```python
from build123d import *

# Parameters (mm, degrees)
CUT_EXTRUDE1_START        = 15
CUT_EXTRUDE1_DEPTH        = 10.5
CUT_EXTRUDE1_START_2      = 25.5
CUT_EXTRUDE1_2_DEPTH      = 4
CUT_EXTRUDE1_START_3      = -5
CUT_EXTRUDE1_3_DEPTH      = 3.568757805
BOSS_EXTRUDE1_DEPTH       = 0.5
BOSS_EXTRUDE2_DEPTH       = 0.5
SKETCH4_W                 = 14.5
SKETCH4_H                 = 15
CUT_EXTRUDE2_DEPTH        = 10.672144385
BOSS_EXTRUDE3_DEPTH       = 10.5
F_3_CLEARANCE_HOLE1_D     = 2.9
F_3_CLEARANCE_HOLE1_DEPTH = 6.031783808


with BuildPart() as part:
    # Cut-Extrude1: read off the stored shape, not the designer's step
    # Cut-Extrude1 outline → Cut-Extrude1 (new body)
    with BuildSketch(Plane.XY.offset(CUT_EXTRUDE1_START)):
        with BuildLine():
            Line((337.250458866, -1.431242195), (336.422603251, -1.431242195))
            Line((336.422603251, -1.431242195), (336.422603251, 13.568757805))
            Line((336.422603251, 13.568757805), (323.834138276, 13.568757805))
            Line((323.834138276, 13.568757805), (323.608997572, 10.166078708))
            ThreePointArc((323.608997572, 10.166078708), (323.181382472, 9.560091757), (322.443572772, 9.635667582))
            Line((322.443572772, 9.635667582), (321.491292518, 10.587947835))
            ThreePointArc((321.491292518, 10.587947835), (321.1243382, 10.696161689), (320.834327975, 10.446642593))
            ThreePointArc((320.834327975, 10.446642593), (320.5127775, 9.115460329), (320.529645575, 7.746096829))
            ThreePointArc((320.529645575, 7.746096829), (320.552977781, 7.656046386), (320.596479116, 7.57382043))
            ThreePointArc((320.596479116, 7.57382043), (320.51875348, 5.851708999), (319.722869168, 4.322566357))
            ThreePointArc((319.722869168, 4.322566357), (320.011740784, 3.764617073), (320.636356902, 3.832506086))
            Line((320.636356902, 3.832506086), (321.56122175, 4.617919231))
            ThreePointArc((321.56122175, 4.617919231), (322.32777998, 4.668660807), (322.750458866, 4.027155713))
            Line((322.750458866, 4.027155713), (322.750458866, -4.431242195))
            Line((322.750458866, -4.431242195), (342.750458866, -4.431242195))
            Line((342.750458866, -4.431242195), (342.750458866, -2.431242195))
            Line((342.750458866, -2.431242195), (338.250458866, -2.431242195))
            Line((338.250458866, -2.431242195), (337.250458866, -1.431242195))
        make_face()
    extrude(amount=CUT_EXTRUDE1_DEPTH)

    # Cut-Extrude1 2 outline → Cut-Extrude1 2 (add)
    with BuildSketch(Plane.XY.offset(CUT_EXTRUDE1_START_2)):
        with BuildLine():
            Line((337.250458866, -1.431242195), (336.422603251, -1.431242195))
            Line((336.422603251, -1.431242195), (336.422603251, 13.568757805))
            Line((336.422603251, 13.568757805), (323.834138276, 13.568757805))
            Line((323.834138276, 13.568757805), (323.608997572, 10.166078708))
            ThreePointArc((323.608997572, 10.166078708), (323.181382472, 9.560091757), (322.443572772, 9.635667582))
            Line((322.443572772, 9.635667582), (321.491292518, 10.587947835))
            ThreePointArc((321.491292518, 10.587947835), (321.1243382, 10.696161689), (320.834327975, 10.446642593))
            ThreePointArc((320.834327975, 10.446642593), (320.5127775, 9.115460329), (320.529645575, 7.746096829))
            ThreePointArc((320.529645575, 7.746096829), (320.552977781, 7.656046386), (320.596479116, 7.57382043))
            ThreePointArc((320.596479116, 7.57382043), (320.51875348, 5.851708999), (319.722869168, 4.322566357))
            ThreePointArc((319.722869168, 4.322566357), (320.011740784, 3.764617073), (320.636356902, 3.832506086))
            Line((320.636356902, 3.832506086), (321.56122175, 4.617919231))
            ThreePointArc((321.56122175, 4.617919231), (322.32777998, 4.668660807), (322.750458866, 4.027155713))
            Line((322.750458866, 4.027155713), (322.750458866, -4.431242195))
            Line((322.750458866, -4.431242195), (342.750458866, -4.431242195))
            Line((342.750458866, -4.431242195), (342.750458866, -2.431242195))
            Line((342.750458866, -2.431242195), (338.250458866, -2.431242195))
            Line((338.250458866, -2.431242195), (337.250458866, -1.431242195))
        make_face()
    extrude(amount=CUT_EXTRUDE1_2_DEPTH)

    # Cut-Extrude1 3 outline → Cut-Extrude1 3 (cut)
    with BuildSketch(Plane(origin=(0, 0, 0), x_dir=(1, 0, 0), z_dir=(0, 1, 0)).offset(CUT_EXTRUDE1_START_3)):
        with BuildLine():
            ThreePointArc((336.422603251, -25.5), (337.000458866, -27.5), (336.422603251, -29.5))
            Line((336.422603251, -29.5), (337.750458866, -29.5))
            ThreePointArc((337.750458866, -29.5), (339.750458866, -27.5), (337.750458866, -25.5))
            Line((337.750458866, -25.5), (336.422603251, -25.5))
        make_face()
    extrude(amount=CUT_EXTRUDE1_3_DEPTH, mode=Mode.SUBTRACT)

    # Sketch2 → Boss-Extrude1 (add)
    with BuildSketch(Plane(origin=(0, -2.431242195, 0), x_dir=(-1, 0, 0), z_dir=(0, 1, 0))):
        with BuildLine():
            Line((-338.250458866, 29.5), (-338.250458866, 29.436491673))
            ThreePointArc((-338.250458866, 29.436491673), (-339.750458866, 27.5), (-338.250458866, 25.563508327))
            Line((-338.250458866, 25.563508327), (-338.250458866, 15))
            Line((-338.250458866, 15), (-342.750458866, 15))
            Line((-342.750458866, 15), (-342.750458866, 29.5))
            Line((-342.750458866, 29.5), (-338.250458866, 29.5))
        make_face()
    extrude(amount=BOSS_EXTRUDE1_DEPTH)

    # Sketch3 → Boss-Extrude2 (add)
    with BuildSketch(Plane(origin=(0, -1.931242195, 0), x_dir=(-1, 0, 0), z_dir=(0, 1, 0))):
        with BuildLine():
            Line((-338.250458866, 29.5), (-338.250458866, 29.436491673))
            ThreePointArc((-338.250458866, 29.436491673), (-339.750458866, 27.5), (-338.250458866, 25.563508327))
            Line((-338.250458866, 25.563508327), (-338.250458866, 15))
            Line((-338.250458866, 15), (-342.750458866, 15))
            Line((-342.750458866, 15), (-342.750458866, 29.5))
            Line((-342.750458866, 29.5), (-338.250458866, 29.5))
        make_face()
    extrude(amount=BOSS_EXTRUDE2_DEPTH)

    # Sketch4 → Cut-Extrude2 (cut)
    with BuildSketch(Plane(origin=(336.422603251, 0, 0), x_dir=(0, 0, -1), z_dir=(1, 0, 0))):
        with Locations((-22.25, 6.068757805)):
            Rectangle(SKETCH4_W, SKETCH4_H)
    extrude(amount=-CUT_EXTRUDE2_DEPTH, mode=Mode.SUBTRACT)

    # Sketch5 → Boss-Extrude3 (add)
    with BuildSketch(Plane.XY.offset(29.5)):
        with BuildLine():
            Line((322.750458866, -4.431242195), (322.750458866, 4.027155713))
            ThreePointArc((322.750458866, 4.027155713), (322.32777998, 4.668660807), (321.56122175, 4.617919231))
            Line((321.56122175, 4.617919231), (320.636356902, 3.832506086))
            ThreePointArc((320.636356902, 3.832506086), (320.011740784, 3.764617073), (319.722869168, 4.322566357))
            ThreePointArc((319.722869168, 4.322566357), (320.51875348, 5.851708999), (320.596479116, 7.57382043))
            ThreePointArc((320.596479116, 7.57382043), (320.552977781, 7.656046387), (320.529645575, 7.746096829))
            ThreePointArc((320.529645575, 7.746096829), (320.5127775, 9.11546033), (320.834327975, 10.446642593))
            ThreePointArc((320.834327975, 10.446642593), (321.1243382, 10.696161689), (321.491292518, 10.587947835))
            Line((321.491292518, 10.587947835), (322.443572772, 9.635667582))
            ThreePointArc((322.443572772, 9.635667582), (323.181382472, 9.560091757), (323.608997572, 10.166078708))
            Line((323.608997572, 10.166078708), (323.834138276, 13.568757805))
            Line((323.834138276, 13.568757805), (325.750458866, 13.568757805))
            Line((325.750458866, 13.568757805), (325.750458866, -1.431242195))
            Line((325.750458866, -1.431242195), (337.250458866, -1.431242195))
            Line((337.250458866, -1.431242195), (338.250458866, -2.431242195))
            Line((338.250458866, -2.431242195), (338.250458866, -1.431242195))
            Line((338.250458866, -1.431242195), (342.750458866, -1.431242195))
            Line((342.750458866, -1.431242195), (342.750458866, -4.431242195))
            Line((342.750458866, -4.431242195), (322.750458866, -4.431242195))
        make_face()
    extrude(amount=BOSS_EXTRUDE3_DEPTH)

    # #3 Clearance Hole1
    with Locations(Plane(origin=(325.750458866, 0, 0), x_dir=(0, 0, -1), z_dir=(1, 0, 0))):
        with Locations((-27.5, 7.246096829)):
            Hole(F_3_CLEARANCE_HOLE1_D / 2, depth=F_3_CLEARANCE_HOLE1_DEPTH)


solid = part.part
```
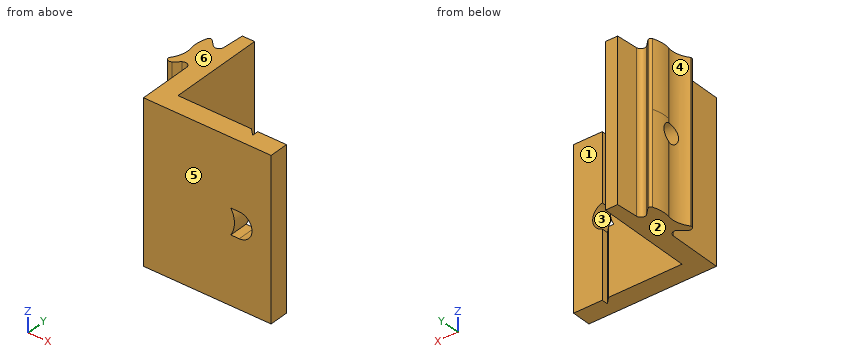
Geometry check sheet. Reference: the model listing, model coordinates, mm. Face numbers are marked on the shaded views. A direction names the side the tool comes from. Give positions to 0.01 mm unless a question says otherwise; leave off trailing zeros. Write each loop counter-clockwise with the first axis right and the second up, starting at its lowest first coordinate (ties: lowest second). Pieces come first, ordered by that corner, then holes. Notation, with made-up numbers: (46, 72.5) - (63, 72.5) arc R14 cw to (63, 82.5) - close; hole circle Ø2 at (-35, 65.5). An arc over 180 degrees is marked (long way). Use a Markdown table: item, result.
Q1. Go/stop test with flat-tipped pins: P1, Ø0.5, axis at y = -2, z = 33, coming from the -X side; P2, Ø3.5, axis at x = 331, z = 24, coming from the +Y side; P3, Ø1.5, axis at x = 328, y = 5, coming from the -Z side; P4, Ø4.5, axis at y = 7.25, z = 27.5, coming from the +X side. Record where each tip stops, or that it passes through.
Computed:
| item | result |
|---|---|
| P1 | stops at x = 322.75 |
| P2 | stops at y = -1.43 |
| P3 | passes through |
| P4 | stops at x = 325.75 |
Q2. Set-up check for the marked faces 1, 2 and 3: record each of +Z, -Z, +X, -X, +Y, -Y from which the full face is reachable in a straight line by a thin tool's end or side.
Computed:
| item | result |
|---|---|
| face 1 | +Z, -Z, +X, +Y |
| face 2 | -Z, +X, -X, +Y, -Y |
| face 3 | +Y, -Y |
Q3. Section check B-B, the plane z = 19.25. Enter the section's corners in (x, y).
Computed:
| item | result |
|---|---|
| outline | (319.72, 4.32) arc R0.56 ccw to (320.64, 3.83) - (321.56, 4.62) arc R0.76 cw to (322.75, 4.03) - (322.75, -4.43) - (342.75, -4.43) - (342.75, -1.43) - (338.25, -1.43) - (338.25, -2.43) - (337.25, -1.43) - (325.75, -1.43) - (325.75, 13.57) - (323.83, 13.57) - (323.61, 10.17) arc R0.73 cw to (322.44, 9.64) - (321.49, 10.59) arc R0.4 ccw to (320.83, 10.45) arc R5.51 ccw to (320.53, 7.75) arc R0.4 ccw to (320.6, 7.57) arc R4 cw to start |
Q4. Draft check along Y on the marked faces 4, 5 and 6. Enter one of: pulls with the +Y half, pulls with the -Y half, needs draft (parallel to the pull), parting line crosses it, or undercut.
Computed:
| item | result |
|---|---|
| face 4 | undercut |
| face 5 | pulls with the -Y half |
| face 6 | needs draft |
Q5. Thickness scan on L1, parallel to Y at x = 324.35, z = 27.5; L2, parallel to Y at x = 323.3, z = 27.5; L3, parallel to X at y = -3.5, z = 36.5. Record the ranges inside material, lowest first. Write a range as [from, to].
Computed:
| item | result |
|---|---|
| L1 | y = [-4.43, 5.8], [8.7, 13.57] |
| L2 | y = [-4.43, 5.8], [8.7, 9.63] |
| L3 | x = [322.75, 342.75] |
Q6. Section check C-C, the plane x = 329. Enter the section's corners in (y, z).
Computed:
| item | result |
|---|---|
| outline | (-4.43, 15) - (-1.43, 15) - (-1.43, 40) - (-4.43, 40) - close |
Q7. Section check A-A, the plane z = 27.5. Enter the section's corners in (x, y).
Computed:
| item | result |
|---|---|
| outline | (319.72, 4.32) arc R0.56 ccw to (320.64, 3.83) - (321.56, 4.62) arc R0.76 cw to (322.75, 4.03) - (322.75, -4.43) - (337, -4.43) - (337, -1.43) - (325.75, -1.43) - (325.75, 5.8) - (320.5, 5.8) arc R4 cw to start; (320.48, 8.7) - (325.75, 8.7) - (325.75, 13.57) - (323.83, 13.57) - (323.61, 10.17) arc R0.73 cw to (322.44, 9.64) - (321.49, 10.59) arc R0.4 ccw to (320.83, 10.45) arc R5.51 ccw to start; (339.75, -4.43) - (342.75, -4.43) - (342.75, -1.43) - (339.75, -1.43) - close |
